from build123d import *

# Parameters (mm, degrees)
SKETCH1_R           = 22.5
SKETCH1_R_2         = 13.5
SKETCH1_W           = 5
SKETCH1_H           = 5
BOSS_EXTRUDE1_DEPTH = 5


with BuildPart() as part:
    # Sketch1 → Boss-Extrude1 (new body)
    with BuildSketch(Plane.XY):
        Circle(SKETCH1_R)
        Circle(SKETCH1_R_2, mode=Mode.SUBTRACT)
        with Locations((0, 17.5)):
            Rectangle(SKETCH1_W, SKETCH1_H, mode=Mode.SUBTRACT)
        Polygon((18.570508076, 7.834936491), (14.240381057, 5.334936491), (11.740381057, 9.665063509), (16.070508076, 12.165063509), align=None, mode=Mode.SUBTRACT)
        Polygon((16.070508076, -12.165063509), (11.740381057, -9.665063509), (14.240381057, -5.334936491), (18.570508076, -7.834936491), align=None, mode=Mode.SUBTRACT)
        with Locations((0, -17.5)):
            Rectangle(SKETCH1_W, SKETCH1_H, mode=Mode.SUBTRACT)
        Polygon((-18.570508076, -7.834936491), (-14.240381057, -5.334936491), (-11.740381057, -9.665063509), (-16.070508076, -12.165063509), align=None, mode=Mode.SUBTRACT)
        Polygon((-16.070508076, 12.165063509), (-11.740381057, 9.665063509), (-14.240381057, 5.334936491), (-18.570508076, 7.834936491), align=None, mode=Mode.SUBTRACT)
    extrude(amount=BOSS_EXTRUDE1_DEPTH)


solid = part.part
The model under review builds one solid part; all positions refer to its coordinate system, in mm. Round coordinates to 2 decimals unless told otherwise and drop trailing zeros. Write each loop counter-clockwise with the first axis right and the second up, starting at its lowest first coordinate (ties: lowest second). Pieces come first, ordered by that corner, then holes. Notation, with made-up numbers: (-18, 59) - (-14, 59) arc R24 ccw to (-14, 73) - close; hole circle Ø6 at (75.25, 71.5). An arc over 180 degrees is marked (long way). One line per item, written item: value. Start each with the question number.
1. Consider section C-C on z = 2.1. Write out the cut boundary in (x, y), and give its area (3 significant figures).
2. Consider section A-A on x = 0. Write out the cut boundary in (y, z), and give its area (3 significant figures).
3. Consider section B-B on y = 0. Write out the cut boundary in (x, z), and give its area (3 significant figures).
4. To check wall thickness, follow L1, parallel to Y at x = 0, z = 2.95; L2, parallel to X at y = 5.5, z = 2.35; L3, parallel to X at y = 10, z = 2.25. State the ranges of each line that lie inside material, in increasing order. Write a range as from..to.
5. Clearance check with flat-ended pins moving along their axes: P1, Ø2.5, axis at y = 17.5, z = 3, coming from the -X side; P2, Ø1.5, axis at x = 0, z = 2.5, coming from the -Y side; P3, Ø1, axis at y = 6, z = 1, coming from the +X side; P4, Ø24.5, axis at x = 0, y = 0, coming from the -Z side. State where each tip first meets the part, or that it passes through.
6. The part is to be moulded in two halves that separate along X. For faces 1 (the face through (0, 20, 2)), 2 (the face through (10.382, -19.961, 2.465)), 3 (the face through (10, -10, 0)), say which applies: released by +X, released by -X, zero draft, split by the parting line, or undercut.
7. Consider section D-D on x = -9. Write out the cut boundary in (y, z), and give its area (3 significant figures).
Checks:
1. outline: circle Ø45 at (0, 0); hole (-18.57, -7.83) - (-16.07, -12.17) - (-11.74, -9.67) - (-14.24, -5.33) - close; hole (-18.57, 7.83) - (-14.24, 5.33) - (-11.74, 9.67) - (-16.07, 12.17) - close; hole circle Ø27 at (0, 0); hole (-2.5, -20) - (2.5, -20) - (2.5, -15) - (-2.5, -15) - close; hole (-2.5, 15) - (2.5, 15) - (2.5, 20) - (-2.5, 20) - close; hole (11.74, -9.67) - (16.07, -12.17) - (18.57, -7.83) - (14.24, -5.33) - close; hole (11.74, 9.67) - (14.24, 5.33) - (18.57, 7.83) - (16.07, 12.17) - close
1. area: 868 mm^2
2. outline: (-22.5, 0) - (-20, 0) - (-20, 5) - (-22.5, 5) - close; (-15, 0) - (-13.5, 0) - (-13.5, 5) - (-15, 5) - close; (13.5, 0) - (15, 0) - (15, 5) - (13.5, 5) - close; (20, 0) - (22.5, 0) - (22.5, 5) - (20, 5) - close
2. area: 40.0 mm^2
3. outline: (-22.5, 0) - (-13.5, 0) - (-13.5, 5) - (-22.5, 5) - close; (13.5, 0) - (22.5, 0) - (22.5, 5) - (13.5, 5) - close
3. area: 90.0 mm^2
4. L1: y = -22.5..-20, -15..-13.5, 13.5..15, 20..22.5
4. L2: x = -21.82..-14.53, -14.15..-12.33, 12.33..14.15, 14.53..21.82
4. L3: x = -20.16..-17.32, -12.32..-9.07, 9.07..12.32, 17.32..20.16
5. P1: stops at x = -15.56
5. P2: stops at y = -22.5
5. P3: stops at x = 21.82
5. P4: passes through
6. face 1: undercut
6. face 2: split by the parting line
6. face 3: zero draft
7. outline: (-20.62, 0) - (-10.06, 0) - (-10.06, 5) - (-20.62, 5) - close; (10.06, 0) - (20.62, 0) - (20.62, 5) - (10.06, 5) - close
7. area: 106 mm^2
